from build123d import *

# Parameters (mm, degrees)
TOP_PROFILE_W                  = 139.7
TOP_PROFILE_H                  = 6.35
WALL_MID_DEPTH                 = 31.75
F_3_0MM_DOWEL_HOLE1_D          = 3
MOTOR_INTERFERECNE_DEPTH       = 3.81
FILLET2_R                      = 5.08
F_3_0MM_DOWEL_HOLE2_AT_2_COUNT = 2
F_3_0MM_DOWEL_HOLE2_AT_2_PITCH = 19.05
F_3_0MM_DOWEL_HOLE4_D          = 3
F_3_0MM_DOWEL_HOLE4_DEPTH      = 6.35
F_3_0MM_DOWEL_HOLE4_TIP        = 0.901290929


with BuildPart() as part:
    # top profile → wall mid (new body)
    with BuildSketch(Plane(origin=(0, 0, 0), x_dir=(1, 0, 0), z_dir=(0, 1, 0))):
        with Locations((69.85, -3.175)):
            Rectangle(TOP_PROFILE_W, TOP_PROFILE_H)
    extrude(amount=WALL_MID_DEPTH)

    # Ø3.0mm Dowel Hole1 (through all)
    with Locations(Plane(origin=(0, 0, 0), x_dir=(1, 0, 0), z_dir=(0, 0, -1))):
        with Locations((38.1, -6.35), (38.1, -25.4)):
            Hole(F_3_0MM_DOWEL_HOLE1_D / 2)

    # Sketch8 → motor interferecne (cut)
    with BuildSketch(Plane.XY):
        Polygon((10.16, 28.575), (35.56, 28.575), (35.56, 20.955), (38.1, 20.955), (38.1, 10.795), (35.56, 10.795), (35.56, 3.175), (10.16, 3.175), align=None)
    extrude(amount=MOTOR_INTERFERECNE_DEPTH, mode=Mode.SUBTRACT)

    # Fillet2
    # the kernel refuses this fillet: 5.08 mm, written as the material it adds along each edge
    with BuildSketch(Plane(origin=(10.16, 3.175, 0), x_dir=(1, 0, 0), z_dir=(0, 0, 1)), Plane(origin=(35.56, 3.175, 0), x_dir=(0, 1, 0), z_dir=(0, 0, 1)), Plane(origin=(35.56, 28.575, 0), x_dir=(-1, 0, 0), z_dir=(0, 0, 1))) as fillet2_piece_1:
        with BuildLine():
            CenterArc((FILLET2_R, FILLET2_R), FILLET2_R, 180, 90)
            Line((0, FILLET2_R), (-FILLET2_R * 0.02, FILLET2_R))
            Line((-FILLET2_R * 0.02, FILLET2_R), (-FILLET2_R * 0.02, -FILLET2_R * 0.02))
            Line((-FILLET2_R * 0.02, -FILLET2_R * 0.02), (FILLET2_R, -FILLET2_R * 0.02))
            Line((FILLET2_R, -FILLET2_R * 0.02), (FILLET2_R, 0))
        make_face()
    extrude(amount=3.81)
    with BuildSketch(Plane(origin=(10.16, 28.575, 0), x_dir=(1, 0, 0), z_dir=(0, 0, 1))) as fillet2_piece_2:
        with BuildLine():
            CenterArc((FILLET2_R, -FILLET2_R), FILLET2_R, 90, 90)
            Line((0, -FILLET2_R), (-FILLET2_R * 0.02, -FILLET2_R))
            Line((-FILLET2_R * 0.02, -FILLET2_R), (-FILLET2_R * 0.02, FILLET2_R * 0.02))
            Line((-FILLET2_R * 0.02, FILLET2_R * 0.02), (FILLET2_R, FILLET2_R * 0.02))
            Line((FILLET2_R, FILLET2_R * 0.02), (FILLET2_R, 0))
        make_face()
    extrude(amount=3.81)
    with BuildSketch(Plane(origin=(38.1, 10.795, 0), x_dir=(0, 1, 0), z_dir=(0, 0, 1))) as fillet2_piece_3:
        with BuildLine():
            CenterArc((4.399409051, 5.08), FILLET2_R, 210, 60)
            Line((0, 2.54), (-0.087988181, 2.4892))
            ThreePointArc((-0.087988181, 2.4892), (-0.1016, 1.27), (-0.1016, 0))
            Line((-0.1016, 0), (0, -0.1016))
            Line((0, -0.1016), (4.399409051, -0.1016))
            Line((4.399409051, -0.1016), (4.399409051, 0))
        make_face()
    extrude(amount=3.81)
    with BuildSketch(Plane(origin=(38.1, 20.955, 0), x_dir=(-1, 0, 0), z_dir=(0, 0, 1))) as fillet2_piece_4:
        with BuildLine():
            CenterArc((5.08, 4.399409051), FILLET2_R, 180, 60)
            Line((0, 4.399409051), (-0.1016, 4.399409051))
            Line((-0.1016, 4.399409051), (-0.1016, 0))
            Line((-0.1016, 0), (0, -0.1016))
            ThreePointArc((0, -0.1016), (1.27, -0.1016), (2.4892, -0.087988181))
            Line((2.4892, -0.087988181), (2.54, 0))
        make_face()
    extrude(amount=3.81)

    # Sketch13 → Ø3.0mm Dowel Hole2 (revolve, cut)
    with BuildSketch(Plane(origin=(0, 25.4, 3.175), x_dir=(0, 0, 1), z_dir=(0, 1, 0))):
        Polygon((0, 0), (0, 8.521290929), (1.5, 7.62), (1.5, 0), align=None)
    f_3_0mm_dowel_hole2 = revolve(axis=Axis((-6.35, 25.4, 3.175), (1, 0, 0)), mode=Mode.SUBTRACT)

    # Ø3.0mm Dowel Hole2 at 2: Ø3.0mm Dowel Hole2 ×2
    with Locations(*[(0, -i * F_3_0MM_DOWEL_HOLE2_AT_2_PITCH, 0) for i in range(1, F_3_0MM_DOWEL_HOLE2_AT_2_COUNT)]):
        add(f_3_0mm_dowel_hole2, mode=Mode.SUBTRACT)

    # Mirror1: Ø3.0mm Dowel Hole2 across plane
    add(f_3_0mm_dowel_hole2.mirror(Plane.ZY.offset(-69.85)), mode=Mode.SUBTRACT)

    # Mirror1 copy 1 sketch → Mirror1 copy 1 (revolve, cut)
    with BuildSketch(Plane(origin=(139.7, 6.35, 3.175), x_dir=(0, 0, 1), z_dir=(0, 1, 0))):
        Polygon((0, 0), (0, -8.521290929), (1.5, -7.62), (1.5, 0), align=None)
    revolve(axis=Axis((146.05, 6.35, 3.175), (1, 0, 0)), mode=Mode.SUBTRACT)

    # Ø3.0mm Dowel Hole4
    with Locations(Plane(origin=(146.05, 31.75, -25.4), x_dir=(-1, 0, 0), z_dir=(0, 1, 0))):
        with Locations((26.35, 28.575), (100.65, 28.575)):
            Hole(F_3_0MM_DOWEL_HOLE4_D / 2, depth=F_3_0MM_DOWEL_HOLE4_DEPTH)
            with Locations((0, 0, -(F_3_0MM_DOWEL_HOLE4_DEPTH + F_3_0MM_DOWEL_HOLE4_TIP / 2))):  # 118° drill point
                Cone(0, F_3_0MM_DOWEL_HOLE4_D / 2, F_3_0MM_DOWEL_HOLE4_TIP, mode=Mode.SUBTRACT)


solid = part.part
Read the model definition and answer for the solid it produces. Units are mm, in the model's axes. A direction names the side the tool comes from. Coordinates: 2 decimals unless noted, no trailing zeros. Loops run counter-clockwise (first coordinate to the right, second up) from the corner with the lowest first, then second, coordinate; pieces in that order, holes last.
Q1. The part is cut by section A-A on x = 13. Write down the section's boundary in (y, z), and give its area (3 significant figures).
Q2. Consider probe 1 along Z at (x, y) = (3.5, 25.4) (3 decimals); probe 2 along X at (y, z) = (16, 0.5); probe 3 along Y at (x, z) = (133.5, 2). Determine where each line is inside the solid, lowest interval first.
Q3. Which of the six approach directions +Z, -Z, +X, -X, +Y, -Y give full straight-line access (tool end or side, diameter ignored) to faces 5 (the face through (34.11, 27.05, 1.88)), 6 (the face through (135.943, 4.863, 2.98)), 7 (the face through (36.67, 24.95, 3.22)), 8 (the face through (3.757, 5.336, 2.069))?
Q4. The mould has two halves that part along X. Classify faces 1 (the face through (0, 16, 3)), 2 (the face through (135.943, 24.386, 2.069)), 3 (the face through (46.83, 28.53, 3.63)), 4 (the face through (45.152, 24.655, 3.253)): +X half, -X half, draft (parallel to the pull), parting line (faces both ways), or undercut.
Q5. Each of these flat-tipped pins is pushed along its axis until it touches: pin 1 Ø1.5 at (y, z) = (15.5, 1) entering from -X; pin 2 Ø2.5 at (x, y) = (38.1, 6.35) entering from -Z; pin 3 Ø2.5 at (x, z) = (119.7, 3.175) entering from +Y; pin 4 Ø2.5 at (y, z) = (25.4, 3.175) entering from -X. Where does it stop, or does it pass through?
Results below:
1. outline: (0, 0) - (3.7, 0) - (3.7, 3.81) - (28.05, 3.81) - (28.05, 0) - (31.75, 0) - (31.75, 6.35) - (0, 6.35) - close
1. area: 109 mm2
2. probe 1: z = 0 to 1.675, 4.675 to 6.35
2. probe 2: x = 0 to 10.16, 38.1 to 139.7
2. probe 3: y = 0 to 5.42, 7.28 to 24.47, 26.33 to 31.75
3. face 5: -Z
3. face 6: +X
3. face 7: +Z, -Z
3. face 8: -X
4. face 1: -X half
4. face 2: draft
4. face 3: undercut
4. face 4: undercut
5. pin 1: stops at x = 0
5. pin 2: passes through
5. pin 3: stops at y = 25.25
5. pin 4: stops at x = 7.77
